```python
from build123d import *

# Parameters (mm, degrees)
F1_DEPTH = 88.9
F2_R     = 1.92798
F3_DEPTH = 25.4
F4_R     = 1.963554
F5_DEPTH = 25.4


with BuildPart() as f1:
    # F0 (on Front) → F1 (new body)
    with BuildSketch(Plane.XZ):
        Polygon((-37.788483, 47.28636), (-39.553114, 47.28636), (-39.553114, 40.374884), (-36.170904, 40.374884), (-32.788693, 40.374884), (-32.788693, 47.28636), (-34.84743, 47.28636), (-34.994483, 41.84541), (-37.788483, 41.84541), align=None)
    extrude(amount=F1_DEPTH)

    # F2 (on face) → F3 (cut)
    with BuildSketch(Plane(origin=(-39.553114, 0, 0), x_dir=(0, -1, 0), z_dir=(-1, 0, 0))):
        with Locations((5.058136, 44.765752)):
            Circle(F2_R)
    extrude(amount=-F3_DEPTH, mode=Mode.SUBTRACT)

    # F4 (on face) → F5 (cut)
    with BuildSketch(Plane(origin=(-39.553114, 0, 0), x_dir=(0, -1, 0), z_dir=(-1, 0, 0))):
        with Locations((79.155207, 43.916043)):
            Circle(F4_R)
    extrude(amount=-F5_DEPTH, mode=Mode.SUBTRACT)


solid = f1.part
```
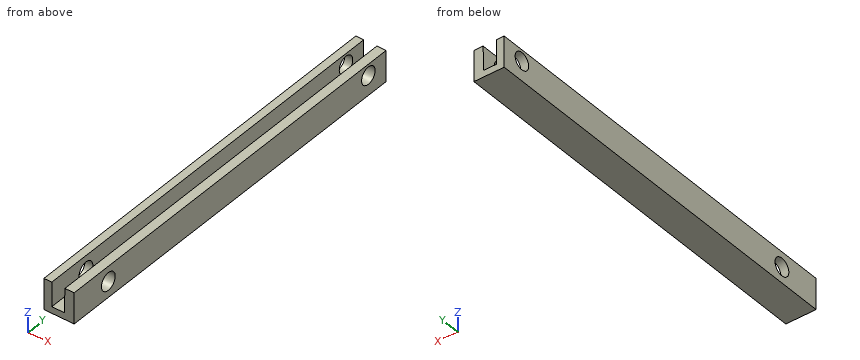
Work out the finished part from the listing and answer in its coordinate system (mm). Give positions to 0.01 mm unless a question says otherwise; leave off trailing zeros. Loops run counter-clockwise (first coordinate to the right, second up) from the corner with the lowest first, then second, coordinate; pieces in that order, holes last. Notation, with made-up numbers: (50, 18) - (54, 18) arc R18 ccw to (54, 47) - close; hole circle Ø6 at (85, -2.5). An arc over 180 degrees is marked (long way). One line per question, with ' | ' between items.
(1) Each of these flat-tipped pins is pushed along its axis until it touches: pin 1 Ø2.5 at (y, z) = (-79.16, 43.92) entering from -X; pin 2 Ø3 at (x, y) = (-36.5, -22.5) entering from +Z. Where does it stop, or does it pass through?
Recorded:
pin 1: passes through | pin 2: stops at z = 47.29
(2) Straight lines are drawn through the part: probe 1 along Y at (x, z) = (-38.75, 43.75); probe 2 along X at (y, z) = (-56, 43.5); probe 3 along Z at (x, y) = (-38.75, -79). For each, find the intervals that lie inside material, in ascending order.
Recorded:
probe 1: y = -88.9 to -81.11, -77.2 to -6.7, -3.42 to 0 | probe 2: x = -39.55 to -37.79, -34.95 to -32.79 | probe 3: z = 40.37 to 41.96, 45.87 to 47.29
(3) The part is cut by section A-A (y = -80). Write down the section's boundary in (x, z), then the cut area to 3 significant figures.
Recorded:
outline: (-39.55, 40.37) - (-32.79, 40.37) - (-32.79, 42.14) - (-34.99, 42.14) - (-34.99, 41.85) - (-37.79, 41.85) - (-37.79, 42.14) - (-39.55, 42.14) - close; (-39.55, 45.69) - (-37.79, 45.69) - (-37.79, 47.29) - (-39.55, 47.29) - close; (-34.89, 45.69) - (-32.79, 45.69) - (-32.79, 47.29) - (-34.85, 47.29) - close | area: 17.3 mm²
(4) The part is cut by section C-C (x = -33.75). Write down the section's boundary in (y, z).
Recorded:
outline: (-88.9, 40.37) - (0, 40.37) - (0, 47.29) - (-88.9, 47.29) - close; hole circle Ø3.93 at (-79.16, 43.92); hole circle Ø3.86 at (-5.06, 44.77)
(5) The part is cut by section B-B (y = -59). Write down the section's boundary in (x, z).
Recorded:
outline: (-39.55, 40.37) - (-32.79, 40.37) - (-32.79, 47.29) - (-34.85, 47.29) - (-34.99, 41.85) - (-37.79, 41.85) - (-37.79, 47.29) - (-39.55, 47.29) - close
